Study the drawing (mm; zero at the part's minimum x, y, z) and answer. Coordinates: 2 decimals unless noted, no trailing zeros. Loops run counter-clockwise (first coordinate to the right, second up) from the corner with the lowest first, then second, coordinate; pieces in that order, holes last. Notation, with made-up numbers: (-13, 75) - (40, 75) arc R25 cw to (40, 99) - close; hole circle Ø4 at (33.25, -7). An arc over 180 degrees is marked (long way). Use one line per item in the form item = value. Start each with the question number.
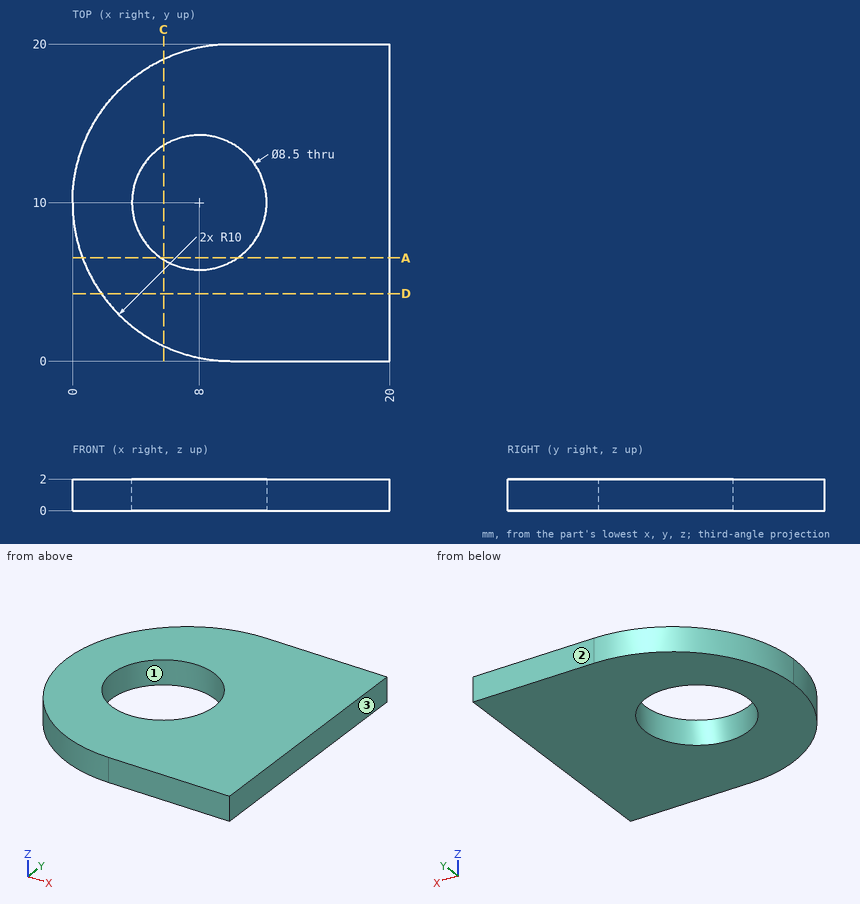
(1) A cutting plane is placed at C-C (x = 5.75). Determine the outline of the cut face in (y, z).
(2) Find the intervals of material crossed by probe 1 along X at (y, z) = (7.5, 0.1); probe 2 along Y at (x, z) = (10.5, 0.1); probe 3 along Y at (x, z) = (8, 1.2), in increasing order. Write a range as from..to.
(3) Each of these flat-tipped pins is pushed along its axis until it touches: pin 1 Ø1.5 at (x, y) = (6, 13) entering from -Z; pin 2 Ø1 at (x, z) = (6.5, 1.5) entering from -Y. Where does it stop, or does it pass through?
(4) Determine the mould class of the marked faces 1, 2 and 3 for opening direction X: +X half, -X half, draft (parallel to the pull), parting line (faces both ways), or undercut.
(5) A cutting plane is placed at D-D (y = 4.25). Determine the outline of the cut face in (x, z).
(6) A cutting plane is placed at A-A (y = 6.5). Determine the outline of the cut face in (x, z), then the cut area to 3 significant figures.
Evaluation:
q1.outline = (0.95, 0) - (6.39, 0) - (6.39, 2) - (0.95, 2) - close; (13.61, 0) - (19.05, 0) - (19.05, 2) - (13.61, 2) - close
q2.probe_1 = 0.32..4.56, 11.44..20
q2.probe_2 = 0..6.56, 13.44..20
q2.probe_3 = 0.2..5.75, 14.25..19.8
q3.pin_1 = 0
q3.pin_2 = 0.46
q4.face_1 = undercut
q4.face_2 = draft
q4.face_3 = +X half
q5.outline = (1.82, 0) - (20, 0) - (20, 2) - (1.82, 2) - close
q6.outline = (0.63, 0) - (5.59, 0) - (5.59, 2) - (0.63, 2) - close; (10.41, 0) - (20, 0) - (20, 2) - (10.41, 2) - close
q6.area = 29.1 mm^2
